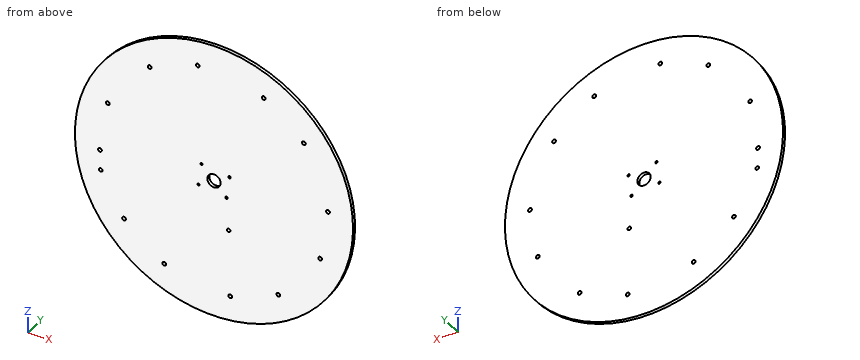
from build123d import *

# Parameters (mm, degrees)
SKETCH2_R               = 125
BOSS_EXTRUDE1_DEPTH     = 3
CUT_EXTRUDE1_START      = -26
SKETCH3_R               = 1.7
CUT_EXTRUDE1_DEPTH      = 88
CUT_EXTRUDE2_DEPTH      = 55
CUT_EXTRUDE2_DEPTH_BACK = 12
SKETCH4_R               = 6
SKETCH5_R               = 1.6
CUT_EXTRUDE3_DEPTH      = 177.802149308
CUT_EXTRUDE4_REACH      = 178.802
SKETCH6_R               = 1.05
CIRPATTERN1_COUNT       = 6


with BuildPart() as part:
    # Sketch2 → Boss-Extrude1 (new body)
    with BuildSketch(Plane(origin=(0, 0, 0), x_dir=(1, 0, 0), z_dir=(0, 1, 0))):
        with Locations(Location((0, 0, 0), (0, 0, 270))):
            Circle(SKETCH2_R)
    extrude(amount=BOSS_EXTRUDE1_DEPTH)

    # Sketch3 → Cut-Extrude1 (cut)
    with BuildSketch(Plane(origin=(0, 3, 0), x_dir=(1, 0, 0), z_dir=(0, 1, 0)).offset(CUT_EXTRUDE1_START)):
        with Locations(Location((57.824361976, 84.994428132, 0), (0, 0, 270))):
            Circle(SKETCH3_R)
        with Locations(Location((14.606066285, 101.75643704, 0), (0, 0, 270))):
            Circle(SKETCH3_R)
        with Locations(Location((44.695152955, -92.574580495, 0), (0, 0, 270))):
            Circle(SKETCH3_R)
        with Locations(Location((80.820626333, -63.527442972, 0), (0, 0, 270))):
            Circle(SKETCH3_R)
        with Locations(Location((-102.519514931, 7.580152362, 0), (0, 0, 270))):
            Circle(SKETCH3_R)
        with Locations(Location((-95.426692618, -38.228994068, 0), (0, 0, 270))):
            Circle(SKETCH3_R)
    cut_extrude1 = extrude(amount=CUT_EXTRUDE1_DEPTH, mode=Mode.SUBTRACT)

    # Sketch4 → Cut-Extrude2 (cut, two sides: drawn at the far end of the back side and taken through both)
    with BuildSketch(Plane(origin=(0, 3, 0), x_dir=(1, 0, 0), z_dir=(0, 1, 0)).offset(-CUT_EXTRUDE2_DEPTH_BACK)):
        with Locations(Location((0, 0, 0), (0, 0, 270))):
            Circle(SKETCH4_R)
    extrude(amount=CUT_EXTRUDE2_DEPTH + CUT_EXTRUDE2_DEPTH_BACK, mode=Mode.SUBTRACT)

    # Sketch5 → Cut-Extrude3 (cut, through all)
    with BuildSketch(Plane.XZ):
        with Locations(Location((-101.778099897, -25.854755487, 0), (0, 0, 270))):
            Circle(SKETCH5_R)
        with Locations(Location((13.216774043, -41.092175458, 0), (0, 0, 270))):
            Circle(SKETCH5_R)
    extrude(amount=-CUT_EXTRUDE3_DEPTH, mode=Mode.SUBTRACT)

    # Sketch6 → Cut-Extrude4 (cut, up to next)
    with BuildSketch(Plane(origin=(0, 3, 0), x_dir=(1, 0, 0), z_dir=(0, 1, 0)), mode=Mode.PRIVATE) as cut_extrude4_sk1:
        with Locations(Location((11.198414604, 11.625148557, 0), (0, 0, 270))):
            Circle(SKETCH6_R)
    cut_extrude4_tool1 = extrude(cut_extrude4_sk1.sketch, amount=-CUT_EXTRUDE4_REACH, mode=Mode.PRIVATE) & part.part
    # Sketch6 → Cut-Extrude4 (cut, up to next)
    with BuildSketch(Plane(origin=(0, 3, 0), x_dir=(1, 0, 0), z_dir=(0, 1, 0)), mode=Mode.PRIVATE) as cut_extrude4_sk2:
        with Locations(Location((13.889158795, -8.300914364, 0), (0, 0, 270))):
            Circle(SKETCH6_R)
    cut_extrude4_tool2 = extrude(cut_extrude4_sk2.sketch, amount=-CUT_EXTRUDE4_REACH, mode=Mode.PRIVATE) & part.part
    # Sketch6 → Cut-Extrude4 (cut, up to next)
    with BuildSketch(Plane(origin=(0, 3, 0), x_dir=(1, 0, 0), z_dir=(0, 1, 0)), mode=Mode.PRIVATE) as cut_extrude4_sk3:
        with Locations(Location((-11.198414604, -11.625148557, 0), (0, 0, 270))):
            Circle(SKETCH6_R)
    cut_extrude4_tool3 = extrude(cut_extrude4_sk3.sketch, amount=-CUT_EXTRUDE4_REACH, mode=Mode.PRIVATE) & part.part
    # Sketch6 → Cut-Extrude4 (cut, up to next)
    with BuildSketch(Plane(origin=(0, 3, 0), x_dir=(1, 0, 0), z_dir=(0, 1, 0)), mode=Mode.PRIVATE) as cut_extrude4_sk4:
        with Locations(Location((-13.889158795, 8.300914364, 0), (0, 0, 270))):
            Circle(SKETCH6_R)
    cut_extrude4_tool4 = extrude(cut_extrude4_sk4.sketch, amount=-CUT_EXTRUDE4_REACH, mode=Mode.PRIVATE) & part.part
    add(cut_extrude4_tool1.solids().sort_by_distance((11.198415, 3, -11.625149))[0], mode=Mode.SUBTRACT)
    add(cut_extrude4_tool2.solids().sort_by_distance((13.889159, 3, 8.300914))[0], mode=Mode.SUBTRACT)
    add(cut_extrude4_tool3.solids().sort_by_distance((-11.198415, 3, 11.625149))[0], mode=Mode.SUBTRACT)
    add(cut_extrude4_tool4.solids().sort_by_distance((-13.889159, 3, -8.300914))[0], mode=Mode.SUBTRACT)

    # CirPattern1: Cut-Extrude1 ×6 about axis
    cirpattern1_axis = Axis((0, 0, 0), (0, 1, 0))
    for i in range(1, CIRPATTERN1_COUNT):
        add(cut_extrude1.rotate(cirpattern1_axis, i * 360 / CIRPATTERN1_COUNT), mode=Mode.SUBTRACT)


solid = part.part
Can you work these out from the model? Positions are in its coordinate system, mm. Coordinates: 2 decimals unless noted, no trailing zeros. Write each loop counter-clockwise with the first axis right and the second up, starting at its lowest first coordinate (ties: lowest second). Pieces come first, ordered by that corner, then holes. Notation, with made-up numbers: M 54,-17.75 L 81,-17.75 A16 ccw 81,9.25 Z; hole C 59.25,-33.75 d7. An arc over 180 degrees is marked long. Use one line per item in the form item = value.
Q1. If we section it at C-C (y = 2.2): State how many separate pieces and enclosed holes the cut face has, then the cut area to 3 significant figures.
Model answer:
separate_pieces = 1
enclosed_holes = 19
area = 48,800 mm^2
Q2. For P1, Ø3, axis at x = 80.82, z = 63.53, coming from the -Y side; P2, Ø1, axis at y = 2, z = -38, coming from the -X side; P3, Ø1.5, axis at x = 20, y = 1.5, coming from the +Z side, each with a flat end and sliding along its axis, tell me the tip position at first contact or that it passes through.
Model answer:
P1 = through
P2 = -119.24
P3 = 123.51
Q3. If we section it at B-B (z = 0): Write out the boundary of the cut face in (x, y).
Model answer:
outline = M -125,0 L -6,0 L -6,3 L -125,3 Z; M 6,0 L 125,0 L 125,3 L 6,3 Z
Q4. If we section it at D-D (x = 35): Write out the boundary of the cut face in (y, z), then the cut area to 3 significant figures.
Model answer:
outline = M 0,-120 L 3,-120 L 3,120 L 0,120 Z
area = 720 mm^2
Q5. If we section it at A-A (x = 0): Write out the boundary of the cut face in (y, z).
Model answer:
outline = M 0,-125 L 3,-125 L 3,-6 L 0,-6 Z; M 0,6 L 3,6 L 3,125 L 0,125 Z
Q6. I need wall thicknesses on line 1 along X through (y, z) = (2, -1); line 2 along X through (y, z) = (0.9, -8.5); line 3 along Z through (x, y) = (14.5, 0.35). Which ranges of each line are inside material? Lowest first, please. Write a range as from..to.
Model answer:
line_1 = -125..-5.92, 5.92..125
line_2 = -124.71..-103.95, -101.09..-14.92, -12.86..124.71
line_3 = -124.16..-103.45, -100.06..-42.05, -40.14..7.45, 9.15..124.16
